```python
from build123d import *

# Parameters (mm, degrees)
F0_R     = 1.5
F1_DEPTH = 6.35
F2_D     = 4


with BuildPart() as f1:
    # F0 (on Front) → F1 (new body)
    with BuildSketch(Plane.XZ):
        Polygon((180, 112.5), (180, 140), (157.5, 140), (157.5, 133.65), (147.5, 133.65), (147.5, 140), (132.5, 140), (132.5, 133.65), (122.5, 133.65), (122.5, 140), (107.5, 140), (107.5, 133.65), (97.5, 133.65), (97.5, 140), (82.5, 140), (82.5, 133.65), (72.5, 133.65), (72.5, 140), (57.5, 140), (57.5, 133.65), (47.5, 133.65), (47.5, 140), (32.5, 140), (32.5, 133.65), (22.5, 133.65), (22.5, 140), (0, 140), (0, 112.5), (6.35, 112.5), (6.35, 102.5), (0, 102.5), (0, 87.5), (6.35, 87.5), (6.35, 77.5), (0, 77.5), (0, 62.5), (6.35, 62.5), (6.35, 52.5), (0, 52.5), (0, 37.5), (6.35, 37.5), (6.35, 27.5), (0, 27.5), (0, 0), (22.5, 0), (22.5, 6.35), (32.5, 6.35), (32.5, 0), (47.5, 0), (47.5, 6.35), (57.5, 6.35), (57.5, 0), (72.5, 0), (72.5, 6.35), (82.5, 6.35), (82.5, 0), (97.5, 0), (97.5, 6.35), (107.5, 6.35), (107.5, 0), (122.5, 0), (122.5, 6.35), (132.5, 6.35), (132.5, 0), (147.5, 0), (147.5, 6.35), (157.5, 6.35), (157.5, 0), (180, 0), (180, 27.5), (173.65, 27.5), (173.65, 37.5), (180, 37.5), (180, 52.5), (173.65, 52.5), (173.65, 62.5), (180, 62.5), (180, 77.5), (173.65, 77.5), (173.65, 87.5), (180, 87.5), (180, 102.5), (173.65, 102.5), (173.65, 112.5), align=None)
        with Locations((50, 22.5)):
            Circle(F0_R, mode=Mode.SUBTRACT)
        with Locations((130, 22.5)):
            Circle(F0_R, mode=Mode.SUBTRACT)
        with Locations((50, 127.5)):
            Circle(F0_R, mode=Mode.SUBTRACT)
        with BuildLine():
            ThreePointArc((30, 102.5), (31.4644660941, 106.0355339059), (35, 107.5))
            Line((35, 107.5), (145, 107.5))
            ThreePointArc((145, 107.5), (148.5355339059, 106.0355339059), (150, 102.5))
            Line((150, 102.5), (150, 47.5))
            ThreePointArc((150, 47.5), (148.5355339059, 43.9644660941), (145, 42.5))
            Line((145, 42.5), (35, 42.5))
            ThreePointArc((35, 42.5), (31.4644660941, 43.9644660941), (30, 47.5))
            Line((30, 47.5), (30, 102.5))
        make_face(mode=Mode.SUBTRACT)
        with Locations((130, 127.5)):
            Circle(F0_R, mode=Mode.SUBTRACT)
    extrude(amount=F1_DEPTH)

    # F2 (through all)
    with Locations(Plane(origin=(0, 0, 0), x_dir=(1, 0, 0), z_dir=(0, 1, 0))):
        with Locations((50, -127.5), (130, -127.5), (130, -22.5), (50, -22.5)):
            Hole(F2_D / 2)


solid = f1.part
```
Part model, mm, in its own coordinate system. A direction names the side the tool comes from. Coordinates: 2 decimals unless noted, no trailing zeros. Order: outer loops, then holes, each group sorted by start corner. A loop starts at its lowest first (then second) coordinate and runs counter-clockwise, first axis right, second up. Notation, with made-up numbers: (48.5, -30) -> (102.5, -30) arc R13 cw to (102.5, -6) -> close; hole circle Ø1 at (-37.5, -20.5). An arc over 180 degrees is marked (long way). Put each result on its own line as item: value. Start each with the question number.
(1) Band-saw the part on A-A (z = 127.5). Give the cut face in (x, y).
(2) Mould opens along Z. For faces 4 (the face through (115, -3, 140)), 5 (the face through (6.35, -3, 108)), 6 (the face through (180, -3, 70)), 7 (the face through (177, -3, 37.5)) say: pulls with the +Z half, pulls with the -Z half, needs draft (parallel to the pull), parting line crosses it, or undercut.
(3) Probe line 1 along Z through (x, y) = (50, -4); line 2 along X through (y, z) = (-2.5, 127.5); line 3 along Z through (x, y) = (78.5, -5). List the from-to ranges inside material, lowest first. Write a range as [from, to].
(4) Band-saw the part on D-D (y = -3.5). Count the separate pieces of the cut face and the enclosed holes in it, then the cut area to 3 significant figures.
(5) Band-saw the part on B-B (x = 75.5). Give the cut face in (y, z).
(6) Pin check, flat tips, straight feed: pin 1 Ø1.9 at (y, z) = (-2.5, 81) entering from -X; pin 2 Ø3 at (x, y) = (47.5, -1) entering from -Z; pin 3 Ø2 at (y, z) = (-3.5, 31) entering from +X; pin 4 Ø3 at (x, z) = (130, 22.5) entering from -Y. Stop position of each tip, or through.
(7) Band-saw the part on C-C (x = 50). Give the cut face in (y, z).
(8) Which spindle directions (+Z, -Z, +X, -X, +Y, -Y) get a long thin tool onto all of the face, cutting with end or side? Do faces 1 (the face through (102, -3, 6.35)), 2 (the face through (3, -3, 102.5)), 3 (the face through (150, -3, 75)). Say none if no direction does.
Determined:
1. outline: (0, -6.35) -> (48, -6.35) -> (48, 0) -> (0, 0) -> close; (52, -6.35) -> (128, -6.35) -> (128, 0) -> (52, 0) -> close; (132, -6.35) -> (180, -6.35) -> (180, 0) -> (132, 0) -> close
2. face 4: pulls with the +Z half
2. face 5: undercut
2. face 6: needs draft
2. face 7: undercut
3. line 1: z = [6.35, 20.5], [24.5, 42.5], [107.5, 125.5], [129.5, 133.65]
3. line 2: x = [0, 48], [52, 128], [132, 180]
3. line 3: z = [6.35, 42.5], [107.5, 133.65]
4. separate pieces: 1
4. enclosed holes: 5
4. area: 16,100 mm²
5. outline: (-6.35, 6.35) -> (0, 6.35) -> (0, 42.5) -> (-6.35, 42.5) -> close; (-6.35, 107.5) -> (0, 107.5) -> (0, 133.65) -> (-6.35, 133.65) -> close
6. pin 1: stops at x = 6.35
6. pin 2: stops at z = 0
6. pin 3: stops at x = 173.65
6. pin 4: passes through
7. outline: (-6.35, 6.35) -> (0, 6.35) -> (0, 20.5) -> (-6.35, 20.5) -> close; (-6.35, 24.5) -> (0, 24.5) -> (0, 42.5) -> (-6.35, 42.5) -> close; (-6.35, 107.5) -> (0, 107.5) -> (0, 125.5) -> (-6.35, 125.5) -> close; (-6.35, 129.5) -> (0, 129.5) -> (0, 133.65) -> (-6.35, 133.65) -> close
8. face 1: -Z, +Y, -Y
8. face 2: -X, +Y, -Y
8. face 3: +Y, -Y
